Work out the finished part from the listing and answer in its coordinate system (mm). A direction names the side the tool comes from. Give positions to 0.01 mm unless a question says otherwise; leave off trailing zeros. Write each loop counter-clockwise with the first axis right and the second up, starting at its lowest first coordinate (ties: lowest second). Pieces come first, ordered by that corner, then holes.
1) Find section B-B (x = -26.5). Determine the outline of the cut face in (y, z).
2) Find section A-A (z = 34). Determine the outline of the cut face in (x, y), plus the area to 3 significant figures.
3) Determine the mould class of faces 4 (the face through (-25, -75, 24.774)), 5 (the face through (30, -150.95, 86.75)), 6 (the face through (-58.715, -18.771, 31.761)) for opening direction Y: pulls with the +Y half, pulls with the -Y half, needs draft (parallel to the pull), parting line crosses it, or undercut.
4) Given pin 1 Ø5 at (x, y) = (12.5, -85) entering from +Z; pin 2 Ø3 at (x, y) = (-11, -102) entering from +Z; pin 3 Ø23 at (x, y) = (-39, -94.5) entering from -Z; pin 4 Ø17.5 at (x, y) = (10, -45) entering from -Z, each flat-ended and moving along its own axis, determine where each tip first touches the part or whether it passes through.
5) Find section D-D (x = -44). Determine the outline of the cut face in (y, z).
6) Find section C-C (y = -35). Determine the outline of the cut face in (x, z).
7) A tool of negligible diameter and unlimited length cuts with its end or side. For faces 1 (the face through (-15, -38.1, -7)), 2 (the face through (10, -75, 37.474)), 3 (the face through (-17.446, -75, 31)), from which of +Z, -Z, +X, -X, +Y, -Y can it reach the whole face along a straight path? Write none if from no direction.
8) Straight lines are drawn through the part: probe 1 along X at (y, z) = (-60.5, 17.5); probe 2 along Z at (x, y) = (-22, -61); probe 3 along Y at (x, z) = (31, -3.5). For each, find the intervals that lie inside material, in ascending order.
```python
from build123d import *

# Parameters (mm, degrees)
F1_DEPTH = 152.4
F2_W     = 76.2
F2_H     = 12.7
F3_DEPTH = 127
F4_R     = 6.35
F5_DEPTH = 11.58917
F6_DEPTH = 12.91644
F7_R     = 38.1
F8_DEPTH = 25.4
F9_R     = 5.08


with BuildPart() as f1:
    # F0 (on Front) → F1 (new body)
    with BuildSketch(Plane.XZ):
        Polygon((-17.445847, 37.4745), (-71.420847, 37.4745), (-71.420847, -13.3255), (42.879153, -13.3255), (42.879153, 88.2745), (17.479153, 88.2745), (17.479153, 37.4745), (1.604153, 37.4745), (1.604153, 24.7745), (17.479153, 24.7745), (17.479153, 12.0745), (-33.320847, 12.0745), (-33.320847, 24.7745), (-17.445847, 24.7745), align=None)
    extrude(amount=F1_DEPTH)

    # F2 (on face) → F3 (cut)
    with BuildSketch(Plane(origin=(-71.420847, 0, 0), x_dir=(0, -1, 0), z_dir=(-1, 0, 0))):
        with Locations((76.2, -6.9755)):
            Rectangle(F2_W, F2_H)
    extrude(amount=-F3_DEPTH, mode=Mode.SUBTRACT)

    # F4 (on face) → F5 (cut)
    with BuildSketch(Plane.XY.offset(37.4745)):
        with Locations((-52.370847, -19.05)):
            Circle(F4_R)
    extrude(amount=-F5_DEPTH, mode=Mode.SUBTRACT)

    # F4 (on face) → F6 (cut)
    with BuildSketch(Plane.XY.offset(37.4745)):
        with Locations((-52.370847, -133.35)):
            Circle(F4_R)
    extrude(amount=-F6_DEPTH, mode=Mode.SUBTRACT)

    # F7 (on face) → F8 (cut)
    with BuildSketch(Plane.YZ.offset(42.879153)):
        with Locations((-76.2, 88.2745)):
            Circle(F7_R)
    extrude(amount=-F8_DEPTH, mode=Mode.SUBTRACT)

    # F9
    f9_edges = [f1.edges().sort_by_distance(p)[0] for p in [
        (30.179153, 0, 88.2745),
        (30.179153, -152.4, 88.2745),
    ]]
    fillet(f9_edges, radius=F9_R)


solid = f1.part
```
Results:
1. outline: (-152.4, -13.33) - (-114.3, -13.33) - (-114.3, -0.63) - (-38.1, -0.63) - (-38.1, -13.33) - (0, -13.33) - (0, 12.07) - (-152.4, 12.07) - close; (-152.4, 24.77) - (0, 24.77) - (0, 37.47) - (-152.4, 37.47) - close
2. outline: (-71.42, -152.4) - (-17.45, -152.4) - (-17.45, 0) - (-71.42, 0) - close; (1.6, -152.4) - (42.88, -152.4) - (42.88, 0) - (1.6, 0) - close; hole circle Ø12.7 at (-52.37, -133.35); hole circle Ø12.7 at (-52.37, -19.05)
2. area: 14,300 mm2
3. face 4: needs draft
3. face 5: pulls with the -Y half
3. face 6: undercut
4. pin 1: stops at z = 37.47
4. pin 2: stops at z = 12.07
4. pin 3: stops at z = -0.63
4. pin 4: stops at z = -13.33
5. outline: (-152.4, -13.33) - (-114.3, -13.33) - (-114.3, -0.63) - (-38.1, -0.63) - (-38.1, -13.33) - (0, -13.33) - (0, 37.47) - (-152.4, 37.47) - close
6. outline: (-71.42, -13.33) - (42.88, -13.33) - (42.88, 88.27) - (17.48, 88.27) - (17.48, 37.47) - (1.6, 37.47) - (1.6, 24.77) - (17.48, 24.77) - (17.48, 12.07) - (-33.32, 12.07) - (-33.32, 24.77) - (-17.45, 24.77) - (-17.45, 37.47) - (-71.42, 37.47) - close
7. face 1: -Z, +X, -X
7. face 2: +Z, -X, +Y, -Y
7. face 3: +Z, +Y, -Y
8. probe 1: x = -71.42 to -33.32, 17.48 to 42.88
8. probe 2: z = -0.63 to 12.07, 24.77 to 37.47
8. probe 3: y = -152.4 to -114.3, -38.1 to 0
